Geometry check sheet. Reference: the model listing, model coordinates, mm. Round coordinates to 2 decimals unless told otherwise and drop trailing zeros. Write each loop counter-clockwise with the first axis right and the second up, starting at its lowest first coordinate (ties: lowest second). Pieces come first, ordered by that corner, then holes. Notation, with made-up numbers: (-29.5, 6) -> (18.5, 6) arc R19 cw to (18.5, 17) -> close; hole circle Ø2 at (-0.75, 28). An arc over 180 degrees is marked (long way). Use a Markdown table: item, result.
```python
from build123d import *

# Parameters (mm, degrees)
SKETCH2_R           = 2.75
BOSS_EXTRUDE2_DEPTH = 3


with BuildPart() as part:
    # Sketch2 → Boss-Extrude2 (new body)
    with BuildSketch(Plane.XY):
        with BuildLine():
            Line((27.74070529, 245.594851313), (27.74070529, 131.5))
            Line((27.74070529, 131.5), (47.74070529, 131.5))
            Line((47.74070529, 131.5), (47.74070529, 56.5))
            Line((47.74070529, 56.5), (27.74070529, 56.5))
            Line((27.74070529, 56.5), (27.74070529, 17.405148687))
            ThreePointArc((27.74070529, 17.405148687), (26.47762478, 13.3410126), (23.133396465, 10.708768028))
            ThreePointArc((23.133396465, 10.708768028), (20.1856831, 8.526218264), (18.792007247, 5.133548935))
            ThreePointArc((18.792007247, 5.133548935), (18.020142632, 2.644369817), (16.409580407, 0.595497692))
            ThreePointArc((16.409580407, 0.595497692), (16.190613984, -11.709412188), (28.464054129, -10.803089717))
            ThreePointArc((28.464054129, -10.803089717), (30.468885152, -9.051370379), (32.974636764, -8.151883342))
            ThreePointArc((32.974636764, -8.151883342), (36.082059553, -6.807278123), (38.161890453, -4.135510355))
            ThreePointArc((38.161890453, -4.135510355), (40.806062267, -1.002196621), (44.734834928, 0.17))
            Line((44.734834928, 0.17), (172.134078399, 0.17))
            ThreePointArc((172.134078399, 0.17), (176.06285106, -1.002196621), (178.707022874, -4.135510355))
            ThreePointArc((178.707022874, -4.135510355), (180.786853774, -6.807278123), (183.894276563, -8.151883342))
            ThreePointArc((183.894276563, -8.151883342), (186.400028175, -9.051370379), (188.404859198, -10.803089717))
            ThreePointArc((188.404859198, -10.803089717), (200.678299343, -11.709412188), (200.45933292, 0.595497692))
            ThreePointArc((200.45933292, 0.595497692), (198.848770695, 2.644369817), (198.076906079, 5.133548935))
            ThreePointArc((198.076906079, 5.133548935), (196.683230227, 8.526218264), (193.735516862, 10.708768028))
            ThreePointArc((193.735516862, 10.708768028), (190.391288547, 13.3410126), (189.128208037, 17.405148687))
            Line((189.128208037, 17.405148687), (189.128208037, 245.594851313))
            ThreePointArc((189.128208037, 245.594851313), (190.391288547, 249.6589874), (193.735516862, 252.291231972))
            ThreePointArc((193.735516862, 252.291231972), (196.683230227, 254.473781736), (198.076906079, 257.866451065))
            ThreePointArc((198.076906079, 257.866451065), (198.848770695, 260.355630183), (200.45933292, 262.404502308))
            ThreePointArc((200.45933292, 262.404502308), (200.678299343, 274.709412188), (188.404859198, 273.803089717))
            ThreePointArc((188.404859198, 273.803089717), (186.400028175, 272.051370379), (183.894276563, 271.151883342))
            ThreePointArc((183.894276563, 271.151883342), (180.786853774, 269.807278123), (178.707022874, 267.135510355))
            ThreePointArc((178.707022874, 267.135510355), (176.06285106, 264.002196621), (172.134078399, 262.83))
            Line((172.134078399, 262.83), (44.734834928, 262.83))
            ThreePointArc((44.734834928, 262.83), (40.806062267, 264.002196621), (38.161890453, 267.135510355))
            ThreePointArc((38.161890453, 267.135510355), (36.082059553, 269.807278123), (32.974636764, 271.151883342))
            ThreePointArc((32.974636764, 271.151883342), (30.468885152, 272.051370379), (28.464054129, 273.803089717))
            ThreePointArc((28.464054129, 273.803089717), (16.190613984, 274.709412188), (16.409580407, 262.404502308))
            ThreePointArc((16.409580407, 262.404502308), (18.020142632, 260.355630183), (18.792007247, 257.866451065))
            ThreePointArc((18.792007247, 257.866451065), (20.1856831, 254.473781736), (23.133396465, 252.291231972))
            ThreePointArc((23.133396465, 252.291231972), (26.47762478, 249.6589874), (27.74070529, 245.594851313))
        make_face()
        with Locations((21.91385104, -5.656854249)):
            Circle(SKETCH2_R, mode=Mode.SUBTRACT)
        with Locations((194.955062287, -5.656854249)):
            Circle(SKETCH2_R, mode=Mode.SUBTRACT)
        with Locations((21.91385104, 268.656854249)):
            Circle(SKETCH2_R, mode=Mode.SUBTRACT)
        with Locations((194.955062287, 268.656854249)):
            Circle(SKETCH2_R, mode=Mode.SUBTRACT)
    extrude(amount=BOSS_EXTRUDE2_DEPTH)


solid = part.part
```
(1) Section check B-B on y = 136. Record the cut outline in (x, z), plus the area to 3 significant figures.
A:
| item | result |
|---|---|
| outline | (27.74, 0) -> (189.13, 0) -> (189.13, 3) -> (27.74, 3) -> close |
| area | 484 mm2 |
(2) Section check C-C on x = 141. Record the cut outline in (y, z).
A:
| item | result |
|---|---|
| outline | (0.17, 0) -> (262.83, 0) -> (262.83, 3) -> (0.17, 3) -> close |
(3) Thickness scan on line 1 (Y direction, x = 167.5, z = 2.15); line 2 (X direction, y = 167, z = 1.55); line 3 (X direction, y = 128.5, z = 0.4). Record the ranges inside material, lowest first.
A:
| item | result |
|---|---|
| line 1 | y = 0.17 to 262.83 |
| line 2 | x = 27.74 to 189.13 |
| line 3 | x = 47.74 to 189.13 |
(4) Section check D-D on z = 1.05. State how many separate pieces and enclosed holes the cut face has, plus the area to 3 significant figures.
A:
| item | result |
|---|---|
| separate pieces | 1 |
| enclosed holes | 4 |
| area | 42,300 mm2 |
(5) Section check A-A on x = 41. Record the cut outline in (y, z), plus the area to 3 significant figures.
A:
| item | result |
|---|---|
| outline | (-0.88, 0) -> (56.5, 0) -> (56.5, 3) -> (-0.88, 3) -> close; (131.5, 0) -> (263.88, 0) -> (263.88, 3) -> (131.5, 3) -> close |
| area | 569 mm2 |
(6) Gauge pin test, flat ends, axial feed: pin 1 Ø1.5 at (y, z) = (111.5, 1) entering from -X; pin 2 Ø0.9 at (x, z) = (38, 2) entering from +Y; pin 3 Ø1.5 at (x, z) = (96.5, 1.5) entering from +Y. Record the tip position at first contact, or that the pin passes through.
A:
| item | result |
|---|---|
| pin 1 | stops at x = 47.74 |
| pin 2 | stops at y = 268.25 |
| pin 3 | stops at y = 262.83 |
(7) Release check for a two-part mould opening along X. For faces 1 (the face through (16.051, -11.575, 1.479)), 2 (the face through (107, 134, 0)), 3 (the face through (200.536, -11.841, 1.479)) record: +X half, -X half, draft (parallel to the pull), parting line (faces both ways), or undercut.
A:
| item | result |
|---|---|
| face 1 | undercut |
| face 2 | draft |
| face 3 | undercut |
